For this review, take the finished solid that the model builds, in its own axes (mm). A direction names the side the tool comes from. Coordinates: 2 decimals unless noted, no trailing zeros. Order: outer loops, then holes, each group sorted by start corner. A loop starts at its lowest first (then second) coordinate and runs counter-clockwise, first axis right, second up. Notation, with made-up numbers: (28, -8.75) - (83, -8.75) arc R33 cw to (83, 26.25) - close; hole circle Ø5 at (-29, -14). An arc over 180 degrees is marked (long way). One line per item, written item: value. Start each with the question number.
(1) Consider section A-A on x = 5.75. Write out the cut boundary in (y, z), then the cut area to 3 significant figures.
(2) Consider section C-C on y = -0.5. Write out the cut boundary in (x, z).
(3) Consider section D-D on y = 18.5. Write out the cut boundary in (x, z).
(4) Consider section B-B on z = -0.75. Write out the cut boundary in (x, y).
(5) To check wall thickness, follow line 1 along Y through (x, z) = (-0.25, 0); line 2 along X through (y, z) = (-9.5, 1); line 3 along Z through (x, y) = (2.5, 3). State the ranges of each line that lie inside material, in increasing order.
(6) Mouldability with a two-part tool opening along Y and no side actions: class faces 1 (the flat face through (0, 22.5, 0)), 2 (the flat face through (12, 0, 0)), 3 (the flat face through (6.35, 0, 0)) as released by +Y, released by -Y, zero draft, split by the parting line, or undercut.
(7) For faces 4 (the flat face through (0, 12.7, 0)), 5 (the cylindrical face through (-11.276, 0.315, 4.736)), list the 3-axis set-ups (+Z, -Z, +X, -X, +Y, -Y) from which the entire face can be reached by the end or side of a thin tool; tool diameter is ignored.
```python
from build123d import *

# Parameters (mm, degrees)
F0_W     = 24
F0_H     = 11
F1_DEPTH = 22.5
F2_R     = 2.54
F3_W     = 12.7
F3_H     = 25.4
F4_DEPTH = 3.683


with BuildPart() as f1:
    # F0 (on Front) → F1 (new body, symmetric)
    with BuildSketch(Plane.XZ):
        Rectangle(F0_W, F0_H)
    extrude(amount=F1_DEPTH, both=True)

    # F2
    f2_edges = [f1.edges().sort_by_distance(p)[0] for p in [
        (-12, 0, 5.5),
        (-12, 0, -5.5),
        (12, 0, -5.5),
        (12, 0, 5.5),
    ]]
    fillet(f2_edges, radius=F2_R)

    # F3 (on Top) → F4 (cut, symmetric)
    with BuildSketch(Plane.XY):
        Rectangle(F3_W, F3_H)
    extrude(amount=F4_DEPTH, both=True, mode=Mode.SUBTRACT)


solid = f1.part
```
Geometry check:
1. outline: (-22.5, -5.5) - (22.5, -5.5) - (22.5, 5.5) - (-22.5, 5.5) - close; hole (-12.7, -3.68) - (12.7, -3.68) - (12.7, 3.68) - (-12.7, 3.68) - close
1. area: 308 mm^2
2. outline: (-12, -2.96) arc R2.54 ccw to (-9.46, -5.5) - (9.46, -5.5) arc R2.54 ccw to (12, -2.96) - (12, 2.96) arc R2.54 ccw to (9.46, 5.5) - (-9.46, 5.5) arc R2.54 ccw to (-12, 2.96) - close; hole (-6.35, -3.68) - (6.35, -3.68) - (6.35, 3.68) - (-6.35, 3.68) - close
3. outline: (-12, -2.96) arc R2.54 ccw to (-9.46, -5.5) - (9.46, -5.5) arc R2.54 ccw to (12, -2.96) - (12, 2.96) arc R2.54 ccw to (9.46, 5.5) - (-9.46, 5.5) arc R2.54 ccw to (-12, 2.96) - close
4. outline: (-12, -22.5) - (12, -22.5) - (12, 22.5) - (-12, 22.5) - close; hole (-6.35, -12.7) - (6.35, -12.7) - (6.35, 12.7) - (-6.35, 12.7) - close
5. line 1: y = -22.5 to -12.7, 12.7 to 22.5
5. line 2: x = -12 to -6.35, 6.35 to 12
5. line 3: z = -5.5 to -3.68, 3.68 to 5.5
6. face 1: released by +Y
6. face 2: zero draft
6. face 3: undercut
7. face 4: none
7. face 5: +Z, -X, +Y, -Y
